Source: CAD feature listing. Evaluate the final solid. Frame: model axes, mm. A direction names the side the tool comes from. Give positions to 0.01 mm unless a question says otherwise; leave off trailing zeros. Loops run counter-clockwise (first coordinate to the right, second up) from the corner with the lowest first, then second, coordinate; pieces in that order, holes last. Notation, with made-up numbers: (-11, -14) -> (-2, -14) arc R24 cw to (-2, 23) -> close; hole circle Ø2 at (14, 75.5). An arc over 180 degrees is marked (long way). Return JSON: item names as keys, results as strings. Group by question number.
```python
from build123d import *
from build123d.topology import SkipClean

# Parameters (mm, degrees)
BOSS_EXTRUDE1_DEPTH     = 25
SKETCH2_W               = 40
SKETCH2_H               = 9
BOSS_EXTRUDE2_DEPTH     = 8.18
FILLET1_R               = 5
CUT_EXTRUDE1_DEPTH      = 47.874168161
CUT_EXTRUDE1_DEPTH_BACK = 47.874168161
SKETCH3_R               = 1.5
SKETCH3_4_R             = 4
CUT_EXTRUDE6_DEPTH      = 47.874168161
SKETCH6_R               = 1.5
CUT_EXTRUDE7_DEPTH      = 48.026142101
CUT_EXTRUDE8_START      = -9
SKETCH6_3_R             = 4
CUT_EXTRUDE8_DEPTH      = 40
FILLET2_R               = 5


with BuildPart() as part:
    # Sketch1 → Boss-Extrude1 (new body)
    with BuildSketch(Plane(origin=(0, 0, 0), x_dir=(1, 0, 0), z_dir=(0, 1, 0))):
        with BuildLine():
            add(Edge.make_bspline(
                [(0, 0), (14.445, 15.64), (28.89, 0)],
                knots=[0, 0, 0, 1, 1, 1], degree=2))
            Line((28.89, 0), (0, 0))
        make_face()
        Polygon((-5.555, -11.82), (34.445, -11.82), (34.445, 0), (28.89, 0), (0, 0), (-5.555, 0), align=None)
    extrude(amount=BOSS_EXTRUDE1_DEPTH)

    # Sketch2 → Boss-Extrude2 (add)
    with BuildSketch(Plane.XY.offset(11.82)):
        with Locations((14.445, 20.5)):
            Rectangle(SKETCH2_W, SKETCH2_H)
    extrude(amount=BOSS_EXTRUDE2_DEPTH)

    # Fillet1
    fillet1_edges = [part.edges().sort_by_distance(p)[0] for p in [
        (14.445, 16, 11.82),
    ]]
    fillet(fillet1_edges, radius=FILLET1_R)

    # Sketch3 → Cut-Extrude1 (cut, two sides: drawn at the far end of the back side and taken through both)
    with BuildSketch(Plane.XY.offset(11.82).offset(-CUT_EXTRUDE1_DEPTH_BACK)):
        with Locations((18.445, 12)):
            Circle(SKETCH3_R)
        with Locations((10.445, 4)):
            Circle(SKETCH3_R)
    extrude(amount=CUT_EXTRUDE1_DEPTH + CUT_EXTRUDE1_DEPTH_BACK, mode=Mode.SUBTRACT)

    # Sketch3<4> → Cut-Extrude6 (cut, through all)
    with SkipClean():  # the faces are left unmerged after this step: merging them gives an invalid solid
        with BuildSketch(Plane.XY.offset(11.82)):
            with Locations((18.445, 12)):
                Circle(SKETCH3_4_R)
        extrude(amount=CUT_EXTRUDE6_DEPTH, mode=Mode.SUBTRACT)

    # Sketch6 → Cut-Extrude7 (cut, through all)
    with SkipClean():  # the faces are left unmerged after this step: merging them gives an invalid solid
        with BuildSketch(Plane(origin=(0, 25, 0), x_dir=(1, 0, 0), z_dir=(0, 1, 0))):
            with Locations(Location((2.445, -16, 0), (0, 0, 270))):
                Circle(SKETCH6_R)
            with Locations(Location((26.445, -16, 0), (0, 0, 270))):
                Circle(SKETCH6_R)
        extrude(amount=-CUT_EXTRUDE7_DEPTH, mode=Mode.SUBTRACT)

    # Sketch6<3> → Cut-Extrude8 (cut)
    with SkipClean():  # the faces are left unmerged after this step: merging them gives an invalid solid
        with BuildSketch(Plane(origin=(0, 25, 0), x_dir=(1, 0, 0), z_dir=(0, 1, 0)).offset(CUT_EXTRUDE8_START)):
            with Locations((2.445, -16)):
                Circle(SKETCH6_3_R)
            with Locations((26.445, -16)):
                Circle(SKETCH6_3_R)
        extrude(amount=-CUT_EXTRUDE8_DEPTH, mode=Mode.SUBTRACT)

    # Fillet2
    fillet2_edges = [part.edges().sort_by_distance(p)[0] for p in [
        (34.445, 20.5, 20),
        (-5.555, 20.5, 20),
    ]]
    fillet(fillet2_edges, radius=FILLET2_R)


solid = part.part
```
1) Reachability of faces 4 (the face through (32, 12, 0)), 5 (the face through (15, 0, 4)) from +Z, -Z, +X, -X, +Y, -Y: full face, straight path, thin tool, end or side. Return the list, or none.
2) Cut plane B-B on y = 20.5. Count the separate pieces of the cut face and the enclosed holes in it, then the cut area to 3 significant figures.
3) Cut plane A-A on z = 16. Return loops of the section in (x, y) (3 decimals), then the cut area to 3 significant figures.
4) Material intervals for line 1 (X direction, y = 4, z = 1.75) (3 decimals); line 2 (X direction, y = 22.5, z = 16) (3 decimals); line 3 (Z direction, x = 31, y = 9.75), sorted ascending.
5) Contact query for flat-ended pins moving along their axis: P1, Ø1.5, axis at x = 25, y = 3, coming from the -Z side; P2, Ø4, axis at x = 18.5, z = 15.5, coming from the -Y side; P3, Ø4, axis at x = 18.445, y = 12, coming from the -Z side; P4, Ø9, axis at x = 2.445, z = 16, coming from the -Y side. Output: stop coordinate, or through.
6) Mould query, pull axis Y, two halves, no side actions, for faces 1 (the face through (-3, 12, 0)), 2 (the face through (14, 16, 17)), 3 (the face through (11.251, 5.265, 1.981)). Classes: released by +Y, released by -Y, zero draft, split by the parting line, or undercut.
Calculated:
{
 "1": {"face 4": "-Z, +X, +Y, -Y", "face 5": "+Z, -Z, +X, -X, -Y"},
 "2": {"separate pieces": "1", "enclosed holes": "2", "area": "926 mm2"},
 "3": {"outline": "(-5.454, 15.932) -> (-1.555, 15.932) -> (-1.555, 16) -> (0.945, 16) -> (0.945, 25) -> (-5.454, 25) -> close; (3.945, 16) -> (6.445, 16) -> (6.445, 15.932) -> (17.712, 15.932) arc R4 cw to (19.178, 15.932) -> (22.445, 15.932) -> (22.445, 16) -> (24.945, 16) -> (24.945, 25) -> (3.945, 25) -> close; (27.945, 16) -> (30.445, 16) -> (30.445, 15.932) -> (34.344, 15.932) -> (34.344, 25) -> (27.945, 25) -> close", "area": "306 mm2"},
 "4": {"line 1": "-5.555 to 8.945, 11.945 to 34.445", "line 2": "-5.454 to 0.945, 3.945 to 24.945, 27.945 to 34.344", "line 3": "0 to 11.82"},
 "5": {"P1": "z = -4.22", "P2": "y = 15.53", "P3": "z = -7.67", "P4": "y = 0"},
 "6": {"face 1": "zero draft", "face 2": "released by -Y", "face 3": "undercut"}
}
